```python
from build123d import *

# Parameters (mm, degrees)
BOSS_EXTRUDE1_DEPTH    = 3
BOSS_EXTRUDE1_TAPER    = 19.5
BOSS_EXTRUDE2_START    = -3
SKETCH3_R              = 9
BOSS_EXTRUDE2_DEPTH    = 20
SKETCH4_R              = 6
CUT_EXTRUDE1_DEPTH     = 10
M12_TAPPED_HOLE1_D     = 10.2
FILLET1_R              = 1
FILLET2_R              = 0.5
LPATTERN1_COUNT        = 2
LPATTERN1_PITCH        = 22
FILLET1_OF_LPATTERN1_R = 1
FILLET2_OF_LPATTERN1_R = 0.5


with BuildPart() as part:
    # Sketch1 → Boss-Extrude1 (new body)
    with BuildSketch(Plane(origin=(0, 0, 0), x_dir=(1, 0, 0), z_dir=(0, 1, 0))):
        Polygon((0, 41.528227513), (-35.9645, -20.764113756), (35.9645, -20.764113756), align=None)
    extrude(amount=BOSS_EXTRUDE1_DEPTH, taper=BOSS_EXTRUDE1_TAPER)

    # Sketch3 → Boss-Extrude2 (add)
    with BuildSketch(Plane(origin=(0, 3, 0), x_dir=(1, 0, 0), z_dir=(0, 1, 0)).offset(BOSS_EXTRUDE2_START)):
        with Locations(Location((0, 16.235886244, 0), (0, 0, 270))):
            Circle(SKETCH3_R)
    boss_extrude2 = extrude(amount=-BOSS_EXTRUDE2_DEPTH)

    # Sketch4 → Cut-Extrude1 (cut)
    with BuildSketch(Plane(origin=(0, 3, 0), x_dir=(1, 0, 0), z_dir=(0, 1, 0))):
        with Locations(Location((0, 16.235886244, 0), (0, 0, 270))):
            Circle(SKETCH4_R)
    cut_extrude1 = extrude(amount=-CUT_EXTRUDE1_DEPTH, mode=Mode.SUBTRACT)

    # M12 Tapped Hole1 (through all)
    with Locations(Plane(origin=(0, -20, 0), x_dir=(-1, 0, 0), z_dir=(0, -1, 0))):
        with Locations((0, 16.235886244)):
            m12_tapped_hole1 = Hole(M12_TAPPED_HOLE1_D / 2)

    # Fillet1
    fillet1_edges = [part.edges().sort_by_distance(p)[0] for p in [
        (0, -20, -25.235886244),
    ]]
    fillet(fillet1_edges, radius=FILLET1_R)

    # Fillet2
    fillet2_edges = [part.edges().sort_by_distance(p)[0] for p in [
        (0, 0, -25.235886244),
    ]]
    fillet(fillet2_edges, radius=FILLET2_R)

    # LPattern1: Boss-Extrude2, Cut-Extrude1, M12 Tapped Hole1 ×2
    with Locations(*[(0, 0, i * LPATTERN1_PITCH) for i in range(1, LPATTERN1_COUNT)]):
        add(boss_extrude2)
        add(cut_extrude1, mode=Mode.SUBTRACT)
        add(m12_tapped_hole1, mode=Mode.SUBTRACT)

    # Fillet1 of LPattern1
    fillet1_of_lpattern1_edges = [part.edges().sort_by_distance(p)[0] for p in [
        (0, -20, -3.235886244),
    ]]
    fillet(fillet1_of_lpattern1_edges, radius=FILLET1_OF_LPATTERN1_R)

    # Fillet2 of LPattern1
    fillet2_of_lpattern1_edges = [part.edges().sort_by_distance(p)[0] for p in [
        (0, 0, -3.235886244),
    ]]
    fillet(fillet2_of_lpattern1_edges, radius=FILLET2_OF_LPATTERN1_R)


solid = part.part
```
Source: CAD feature listing. Evaluate the final solid. Frame: model axes, mm. A direction names the side the tool comes from. Give positions to 0.01 mm unless a question says otherwise; leave off trailing zeros. Write each loop counter-clockwise with the first axis right and the second up, starting at its lowest first coordinate (ties: lowest second). Pieces come first, ordered by that corner, then holes.
1. Pull-direction query (X, two-part tool) for faces 1 (the face through (2.7, -9.62, 14.35)), 2 (the face through (1.802, -1.93, 11.487)), 3 (the face through (10, 0, 5)); classes: +X half, -X half, draft (parallel to the pull), parting line (faces both ways), or undercut.
2. Access query for faces 4 (the face through (2.742, -13.409, 1.464)), 5 (the face through (-5, -7, -18)), 6 (the face through (2.7, -9.62, -7.65)). Directions: +Z, -Z, +X, -X, +Y, -Y. A direction counts if a zero-diameter tool reaches every point of the face in a straight line with its end or side. Return the directions, or none.
3. Section query B-B (y = -17.25). Return the cut outline in (x, z), then the cut area to 3 significant figures.
4. First-contact query: pin 1 (3.5 mm diameter, centred on x = -2.5, z = 3, fed in from +Y); pin 2 (9.5 mm diameter, centred on x = 0, z = 5.76, fed in from +Y); pin 3 (5 mm diameter, centred on x = -13.5, z = -23, fed in from -Y); pin 4 (1.5 mm diameter, centred on y = -2.5, z = -7.5, fed in from +X). Flat tips, straight axial feed; report the tip coordinate or a pass-through.
5. Section query A-A (y = -1.5). Return the cut outline in (x, z), then the cut area to 3 significant figures.
6. Material intervals for line 1 along Z through (x, y) = (3, -0.25); line 2 along Z through (x, y) = (3, 2.25); line 3 along X through (y, z) = (-1.25, 5.5), sorted ascending.
Output values:
1. face 1: parting line
1. face 2: undercut
1. face 3: draft
2. face 4: +Y, -Y
2. face 5: +Y
2. face 6: -Y
3. outline: circle Ø18 at (0, -16.24); circle Ø18 at (0, 5.76); hole circle Ø10.2 at (0, -16.24); hole circle Ø10.2 at (0, 5.76)
3. area: 346 mm2
4. pin 1: stops at y = -7
4. pin 2: passes through
4. pin 3: stops at y = 0
4. pin 4: stops at x = 4.15
5. outline: circle Ø18 at (0, -16.24); circle Ø18 at (0, 5.76); hole circle Ø12 at (0, -16.24); hole circle Ø12 at (0, 5.76)
5. area: 283 mm2
6. line 1: z = -24.79 to -21.43, -11.04 to -7.68, -2.79 to 0.57, 10.96 to 14.32
6. line 2: z = -34.74 to -21.43, -11.04 to 0.57, 10.96 to 19.97
6. line 3: x = -9 to -5.99, 5.99 to 9
